Read the model definition and answer for the solid it produces. Units are mm, in the model's axes. A direction names the side the tool comes from. Round coordinates to 2 decimals unless told otherwise and drop trailing zeros. Write each loop counter-clockwise with the first axis right and the second up, starting at its lowest first coordinate (ties: lowest second). Pieces come first, ordered by that corner, then holes. Notation, with made-up numbers: (42.5, 66.25) -> (84.5, 66.25) arc R18 cw to (84.5, 96.25) -> close; hole circle Ø4 at (46, 67.25). An arc over 180 degrees is marked (long way). Return JSON: item names as keys, results as strings. Group by question number.
(1) For faces 1 (the flat face through (0, 0, 3.175)), 2 (the flat face through (0, 25.4, 401)), determine the directions among +Z, -Z, +X, -X, +Y, -Y from which every point of the face is accessible in a straight line to the end or side of a thin tool.
(2) Straight lines are drawn through the part: line 1 (Y direction, x = -1.5, z = 285.5) (3 decimals); line 2 (Z direction, x = -11, y = 10) (3 decimals). For each, find the intervals that lie inside material, in ascending order.
(3) Given pin 1 (8 mm diameter, centred on x = -11.5, y = 6, fed in from -Z); pin 2 (3 mm diameter, centred on x = -7, y = -16.5, fed in from +Z) (3 decimals), each flat-ended and moving along its own axis, determine where each tip first touches the part or whether it passes through.
(4) The mould has two halves that part along X. Classify faces 3 (the flat face through (25.4, 0, 401)), 4 (the flat face through (1.8, -22.5, 812.8)), 5 (the flat face through (0, -22.225, 402)), 6 (the flat face through (0, 22.225, 402)): released by +X, released by -X, zero draft, split by the parting line, or undercut.
(5) A cutting plane is placed at B-B on y = -8. Give the vertices of the cut face in (x, z) (3 decimals), then the cut area to 3 significant figures.
(6) A cutting plane is placed at A-A on z = 224. Give the vertices of the cut face in (x, y) (3 decimals).
```python
from build123d import *

# Parameters (mm, degrees)
F1_DEPTH = 812.8
F2_T     = 3.175


# Not quite as in the source:
# - a shell that OpenCascade refuses in one call is made with other operations: the cavity is built on its own and cut out


with BuildPart() as f1:
    # F0 (on Top) → F1 (new body)
    with BuildSketch(Plane.XY):
        with BuildLine():
            Line((22.225, 25.4), (-22.225, 25.4))
            ThreePointArc((-22.225, 25.4), (-24.4700640303, 24.4700640303), (-25.4, 22.225))
            Line((-25.4, 22.225), (-25.4, -22.225))
            ThreePointArc((-25.4, -22.225), (-24.4700640303, -24.4700640303), (-22.225, -25.4))
            Line((-22.225, -25.4), (22.225, -25.4))
            ThreePointArc((22.225, -25.4), (24.4700640303, -24.4700640303), (25.4, -22.225))
            Line((25.4, -22.225), (25.4, 22.225))
            ThreePointArc((25.4, 22.225), (24.4700640303, 24.4700640303), (22.225, 25.4))
        make_face()
    extrude(amount=F1_DEPTH)

    # F2: shell of thickness 3.175, made by hand


with BuildPart() as f2_core1:
    # F2_t2: copy of F1
    add(f1.part)

    # the walls: a layer under each face that stays
    f2_faces = [f2_core1.faces().sort_by_distance(p)[0] for p in [
        (0, 25.4, 406.4),
        (-25.4, 0, 406.4),
        (0, -25.4, 406.4),
        (25.4, 0, 406.4),
        (0, 0, 0),
    ]]
    thicken(f2_faces, amount=-F2_T, mode=Mode.SUBTRACT)


with BuildPart() as f1_1:
    add(f1.part)

    # what is left inside the walls is the cavity
    f2_cavity = [f2_core1.part.solids().sort_by_distance(p)[0] for p in [
        (0, 22.19325, 542.925),
    ]]
    add(f2_cavity, mode=Mode.SUBTRACT)


solid = f1_1.part
```
Checks:
{
 "1": {"face 1": "+Z", "face 2": "+Z, -Z, +X, -X, +Y"},
 "2": {"line 1": "y = -25.4 to -22.225, 22.225 to 25.4", "line 2": "z = 0 to 3.175"},
 "3": {"pin 1": "stops at z = 0", "pin 2": "stops at z = 3.175"},
 "4": {"face 3": "released by +X", "face 4": "zero draft", "face 5": "undercut", "face 6": "undercut"},
 "5": {"outline": "(-25.4, 0) -> (25.4, 0) -> (25.4, 812.8) -> (22.225, 812.8) -> (22.225, 3.175) -> (-22.225, 3.175) -> (-22.225, 812.8) -> (-25.4, 812.8) -> close", "area": "5,300 mm^2"},
 "6": {"outline": "(-25.4, -22.225) arc R3.175 ccw to (-22.225, -25.4) -> (22.225, -25.4) arc R3.175 ccw to (25.4, -22.225) -> (25.4, 22.225) arc R3.175 ccw to (22.225, 25.4) -> (-22.225, 25.4) arc R3.175 ccw to (-25.4, 22.225) -> close; hole (-22.225, -22.225) -> (22.225, -22.225) -> (22.225, 22.225) -> (-22.225, 22.225) -> close"}
}
